from build123d import *

# Parameters (mm, degrees)
F0_W     = 25.4
F0_H     = 50.8
F1_DEPTH = 6.35
F2_W     = 6.35
F2_H     = 50.8
F3_DEPTH = 3.175
F4_R     = 2.0193
F5_DEPTH = 6.351


with BuildPart() as f1:
    # F0 (on Front) → F1 (new body)
    with BuildSketch(Plane.XZ):
        Rectangle(F0_W, F0_H)
    extrude(amount=F1_DEPTH)

    # F2 (on face) → F3 (cut)
    with BuildSketch(Plane.XZ.offset(6.35)):
        with Locations((-9.525, 0)):
            Rectangle(F2_W, F2_H)
        with Locations((9.525, 0)):
            Rectangle(F2_W, F2_H)
    extrude(amount=-F3_DEPTH, mode=Mode.SUBTRACT)

    # F4 (on face) → F5 (cut, through all)
    with BuildSketch(Plane.XZ.offset(6.35)):
        Circle(F4_R)
        with Locations((0, 19.05)):
            Circle(F4_R)
        with Locations((0, -19.05)):
            Circle(F4_R)
    extrude(amount=-F5_DEPTH, mode=Mode.SUBTRACT)


solid = f1.part
Geometry: final body of the model. Coordinates: model frame, mm. A direction names the side the tool comes from. Coordinates: 2 decimals unless noted, no trailing zeros. Loops run counter-clockwise (first coordinate to the right, second up) from the corner with the lowest first, then second, coordinate; pieces in that order, holes last. Notation, with made-up numbers: M 51.5,89.25 L 66.5,89.25 A28 cw 66.5,121.25 Z; hole C 72.5,-3 d4. An arc over 180 degrees is marked long. One line per item, written item: value. Start each with the question number.
1) Draft query along Z for faces 4 (the cylindrical face through (-0.263, -3.219, -17.048)), 5 (the flat face through (0, -2, -25.4)), 6 (the flat face through (3, 0, 0)). Return one class per face: released by +Z, released by -Z, zero draft, split by the parting line, or undercut.
2) Cut plane B-B (x = 0). Return loops of the section in (y, z).
3) Cut plane C-C (y = -4.5). Return loops of the section in (x, z), then the cut area to 3 significant figures.
4) Pin query (flat end, axial travel): P1, Ø2.5, axis at y = -5.5, z = 11, coming from the +X side; P2, Ø7, axis at x = -10, z = -7.5, coming from the -Y side (3 decimals); P3, Ø2.5, axis at y = -5, z = 3, coming from the -X side. Return the tip coordinate at first contact, or that it passes through.
5) Cut plane A-A (z = 19.05). Return loops of the section in (x, y) (3 decimals).
6) Cut plane D-D (z = -16.5). Return loops of the section in (x, y) (3 decimals), then the cut area to 3 significant figures.
7) Reachability of faces 1 (the flat face through (6.35, -5, 0)), 2 (the flat face through (0, -2, 25.4)), 3 (the flat face through (-10, -3.175, 0)) from +Z, -Z, +X, -X, +Y, -Y: full face, straight path, thin tool, end or side. Return the list, or none.
8) Material intervals for L1, parallel to Z at x = 0, y = -2.5; L2, parallel to Y at x = -7, z = -15.5 (3 decimals); L3, parallel to X at y = -4.25, z = 6, sorted ascending. Write a range as from..to.
Evaluation:
1. face 4: undercut
1. face 5: released by -Z
1. face 6: zero draft
2. outline: M -6.35,-25.4 L 0,-25.4 L 0,-21.07 L -6.35,-21.07 Z; M -6.35,-17.03 L 0,-17.03 L 0,-2.02 L -6.35,-2.02 Z; M -6.35,2.02 L 0,2.02 L 0,17.03 L -6.35,17.03 Z; M -6.35,21.07 L 0,21.07 L 0,25.4 L -6.35,25.4 Z
3. outline: M -6.35,-25.4 L 6.35,-25.4 L 6.35,25.4 L -6.35,25.4 Z; hole C 0,-19.05 d4.04; hole C 0,0 d4.04; hole C 0,19.05 d4.04
3. area: 607 mm^2
4. P1: x = 6.35
4. P2: y = -3.175
4. P3: x = -6.35
5. outline: M -12.7,-3.175 L -6.35,-3.175 L -6.35,-6.35 L -2.019,-6.35 L -2.019,0 L -12.7,0 Z; M 2.019,-6.35 L 6.35,-6.35 L 6.35,-3.175 L 12.7,-3.175 L 12.7,0 L 2.019,0 Z
6. outline: M -12.7,-3.175 L -6.35,-3.175 L -6.35,-6.35 L 6.35,-6.35 L 6.35,-3.175 L 12.7,-3.175 L 12.7,0 L -12.7,0 Z
6. area: 121 mm^2
7. face 1: +Z, -Z, +X, -Y
7. face 2: +Z, +X, -X, +Y, -Y
7. face 3: +Z, -Z, -X, -Y
8. L1: -25.4..-21.07, -17.03..-2.02, 2.02..17.03, 21.07..25.4
8. L2: -3.175..0
8. L3: -6.35..6.35
